from build123d import *

# Parameters (mm, degrees)
F3_D     = 10.5
F3_DEPTH = 18
F3_TIP   = 3.1545182499
F4_R     = 6.054221828
F5_DEPTH = 14
F6_SIZE  = 0.25


with BuildPart() as f1:
    # F0 (on Right) → F1 (revolve)
    with BuildSketch(Plane.YZ):
        with BuildLine():
            ThreePointArc((16, 0), (3.5916630466, 15.5916630466), (-14.3874945699, 7))
            Line((-14.3874945699, 7), (-16, 7))
            Line((-16, 7), (-19.5, 7))
            Line((-19.5, 7), (-19.5, 0))
            Line((-19.5, 0), (-16, 0))
            Line((-16, 0), (16, 0))
        make_face()
    revolve(axis=Axis((0, 0, 0), (0, 1, 0)))

    # F3
    with Locations(Plane.XZ.offset(19.5)):
        with Locations((0, 0)):
            Hole(F3_D / 2, depth=F3_DEPTH)
            with Locations((0, 0, -(F3_DEPTH + F3_TIP / 2))):  # 118° drill point
                Cone(0, F3_D / 2, F3_TIP, mode=Mode.SUBTRACT)

    # F4 (on face) → F5 (cut)
    with BuildSketch(Plane.XZ.offset(19.5)):
        Circle(F4_R)
    extrude(amount=-F5_DEPTH, mode=Mode.SUBTRACT)

    # F6
    f6_edges = [f1.edges().sort_by_distance(p)[0] for p in [
        (0, -19.5, -7),
        (-6.054222, -19.5, 0),
    ]]
    chamfer(f6_edges, length=F6_SIZE)


solid = f1.part
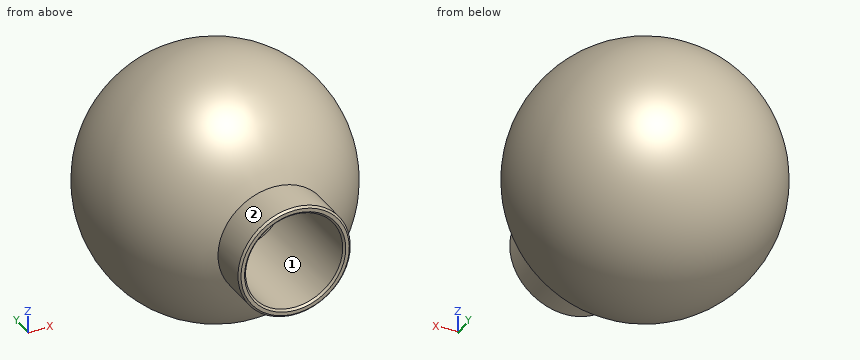
CAD build for the part. Positions are in the model's coordinates, mm. Face numbers are marked on the shaded views. Round coordinates to 2 decimals unless told otherwise and drop trailing zeros. Write each loop counter-clockwise with the first axis right and the second up, starting at its lowest first coordinate (ties: lowest second). Pieces come first, ordered by that corner, then holes. Notation, with made-up numbers: M 41,21.25 L 84,21.25 A12 ccw 84,38.25 Z; hole C -15.75,40.25 d10. An arc over 180 degrees is marked long. Put each result on its own line as item: value. Start each with the question number.
1) Saw through at C-C, the plane x = 8.5. Write the cut outline in (y, z), and give its area (3 significant figures).
2) Saw through at A-A, the plane y = -5. Write the cut outline in (x, z), and give its area (3 significant figures).
3) Pull direction X, two halves, no side cores. Call the marked faces 1 and 2: pulls with the +X half, pulls with the -X half, needs draft (parallel to the pull), parting line crosses it, or undercut.
4) Drill centre lines: probe 1 along X at (y, z) = (-3.3, 0); probe 2 along Z at (x, y) = (0, -3.45); probe 3 along X at (y, z) = (-8, -1.5). Where is each one in solid material? Low to high. Write a range as [from, to].
5) Saw through at B-B, the plane z = 10. Write the cut outline in (x, y).
6) Pin check, flat tips, straight feed: pin 1 Ø3.5 at (x, z) = (2, 3) entering from -Y; pin 2 Ø5 at (y, z) = (-3, -7.5) entering from +X; pin 3 Ø10 at (x, z) = (8.5, 11.5) entering from -Y. Stop position of each tip, or through.
7) Saw through at D-D, the plane y = -15. Write the cut outline in (x, z).
Resolved:
1. outline: C 0,0 d27.11
1. area: 577 mm²
2. outline: C 0,0 d30.4; hole C 0,0 d10.5
2. area: 639 mm²
3. face 1: undercut
3. face 2: parting line crosses it
4. probe 1: [-15.66, -5.25], [5.25, 15.66]
4. probe 2: [-15.62, -5.25], [5.25, 15.62]
4. probe 3: [-13.77, -5.87], [5.87, 13.77]
5. outline: C 0,0 d24.98
6. pin 1: y = -5.5
6. pin 2: x = 15
6. pin 3: y = -13.02
7. outline: C 0,0 d14; hole C 0,0 d12.11
